Input: part model. Units: mm. Frame: model coordinates. Face numbers are marked on the shaded views. A direction names the side the tool comes from. Round coordinates to 2 decimals unless told otherwise and drop trailing zeros. Loops run counter-clockwise (first coordinate to the right, second up) from the corner with the lowest first, then second, coordinate; pieces in that order, holes last. Notation, with made-up numbers: (83, 77.25) -> (112, 77.25) arc R19 ccw to (112, 86.25) -> close; hole circle Ø6 at (39.5, -27). An arc over 180 degrees is marked (long way). One line per question, with ' | ' between items. Start each with the question number.
Q1. Cut plane D-D on y = 58. Return loops of the section in (x, z).
Q2. Cut plane C-C on z = 4.75. State how many separate pieces and enclosed holes the cut face has, and give its area (3 significant figures).
Q3. Cut plane A-A on x = -30. Return loops of the section in (y, z), and give its area (3 significant figures).
Q4. Access query for the marked faces 1, 2 and 3. Directions: +Z, -Z, +X, -X, +Y, -Y. A direction counts if a zero-diameter tool reaches every point of the face in a straight line with its end or side. Return the directions, or none.
Q5. Material intervals for L1, parallel to Y at x = 30, z = 4.25; L2, parallel to Y at x = -40, z = 3.25; L3, parallel to Y at x = 54.5, z = 4.5, sorted ascending.
Q6. Cut plane B-B on x = -15. Return loops of the section in (y, z), and give its area (3 significant figures).
Q7. Mould query, pull axis Y, two halves, no side actions, for the marked faces 4, 5 and 6. Classes: pulls with the +Y half, pulls with the -Y half, needs draft (parallel to the pull), parting line crosses it, or undercut.
Q8. Contact query for a flat-ended pin moving along its axis: P1, Ø2, axis at x = 57.5, z = 3.5, coming from the +Y side. Output: stop coordinate, or through.
from build123d import *

# Parameters (mm, degrees)
BOSS_EXTRU_1_DEPTH      = 8
ESQUISSE2_R             = 2.5
ENL_V_MAT_EXTRU_1_DEPTH = 96.859271852
ENL_V_MAT_EXTRU_4_DEPTH = 96.859271852
ESQUISSE5_R             = 2.5
ENL_V_MAT_EXTRU_5_DEPTH = 96.859271852
ENL_V_MAT_EXTRU_6_DEPTH = 96.859271852


with BuildPart() as part:
    # Esquisse1 → Boss.-Extru.1 (new body)
    with BuildSketch(Plane.XY):
        with BuildLine():
            Line((65, 4), (65, 41))
            ThreePointArc((65, 41), (63.828427125, 43.828427125), (61, 45))
            Line((61, 45), (54, 45))
            ThreePointArc((54, 45), (51.171572875, 46.171572875), (50, 49))
            Line((50, 49), (50, 66))
            ThreePointArc((50, 66), (48.828427125, 68.828427125), (46, 70))
            Line((46, 70), (-46, 70))
            ThreePointArc((-46, 70), (-48.828427125, 68.828427125), (-50, 66))
            Line((-50, 66), (-50, 49))
            ThreePointArc((-50, 49), (-51.171572875, 46.171572875), (-54, 45))
            Line((-54, 45), (-61, 45))
            ThreePointArc((-61, 45), (-63.828427125, 43.828427125), (-65, 41))
            Line((-65, 41), (-65, 4))
            ThreePointArc((-65, 4), (-63.828427125, 1.171572875), (-61, 0))
            Line((-61, 0), (61, 0))
            ThreePointArc((61, 0), (63.828427125, 1.171572875), (65, 4))
        make_face()
    extrude(amount=BOSS_EXTRU_1_DEPTH)

    # Esquisse2 → Enlèv. mat.-Extru.1 (cut, through all)
    with BuildSketch(Plane.XY.offset(8)):
        with Locations((30, 50)):
            Circle(ESQUISSE2_R)
        with Locations(Location((-30, 50, 0), (0, 0, 180))):
            Circle(ESQUISSE2_R)
    extrude(amount=-ENL_V_MAT_EXTRU_1_DEPTH, mode=Mode.SUBTRACT)

    # Esquisse4 → Enlèv. mat.-Extru.4 (cut, through all)
    with BuildSketch(Plane.XY.offset(8)):
        with BuildLine():
            Line((-41, 45), (-10.363961031, 45))
            ThreePointArc((-10.363961031, 45), (-8.978141732, 44.074025149), (-9.303300859, 42.439339828))
            Line((-9.303300859, 42.439339828), (-20.863961031, 30.878679656))
            ThreePointArc((-20.863961031, 30.878679656), (-21.837231077, 30.228361402), (-22.985281374, 30))
            Line((-22.985281374, 30), (-41, 30))
            ThreePointArc((-41, 30), (-42.060660172, 30.439339828), (-42.5, 31.5))
            Line((-42.5, 31.5), (-42.5, 43.5))
            ThreePointArc((-42.5, 43.5), (-42.060660172, 44.560660172), (-41, 45))
        make_face()
        with BuildLine():
            Line((-41, 12), (-10.363961031, 12))
            ThreePointArc((-10.363961031, 12), (-8.978141732, 12.925974851), (-9.303300859, 14.560660172))
            Line((-9.303300859, 14.560660172), (-20.863961031, 26.121320344))
            ThreePointArc((-20.863961031, 26.121320344), (-21.837231077, 26.771638598), (-22.985281374, 27))
            Line((-22.985281374, 27), (-41, 27))
            ThreePointArc((-41, 27), (-42.060660172, 26.560660172), (-42.5, 25.5))
            Line((-42.5, 25.5), (-42.5, 13.5))
            ThreePointArc((-42.5, 13.5), (-42.060660172, 12.439339828), (-41, 12))
        make_face()
        with BuildLine():
            Line((42.5, 43.5), (42.5, 31.5))
            ThreePointArc((42.5, 31.5), (42.060660172, 30.439339828), (41, 30))
            Line((41, 30), (22.985281374, 30))
            ThreePointArc((22.985281374, 30), (21.837231077, 30.228361402), (20.863961031, 30.878679656))
            Line((20.863961031, 30.878679656), (9.303300859, 42.439339828))
            ThreePointArc((9.303300859, 42.439339828), (8.978141732, 44.074025149), (10.363961031, 45))
            Line((10.363961031, 45), (41, 45))
            ThreePointArc((41, 45), (42.060660172, 44.560660172), (42.5, 43.5))
        make_face()
        with BuildLine():
            Line((22.985281374, 27), (41, 27))
            ThreePointArc((41, 27), (42.060660172, 26.560660172), (42.5, 25.5))
            Line((42.5, 25.5), (42.5, 13.5))
            ThreePointArc((42.5, 13.5), (42.060660172, 12.439339828), (41, 12))
            Line((41, 12), (10.363961031, 12))
            ThreePointArc((10.363961031, 12), (8.978141732, 12.925974851), (9.303300859, 14.560660172))
            Line((9.303300859, 14.560660172), (20.863961031, 26.121320344))
            ThreePointArc((20.863961031, 26.121320344), (21.837231077, 26.771638598), (22.985281374, 27))
        make_face()
        with BuildLine():
            Line((-3.378679656, 44.121320344), (-16.878679656, 30.621320344))
            ThreePointArc((-16.878679656, 30.621320344), (-17.757359313, 28.5), (-16.878679656, 26.378679656))
            Line((-16.878679656, 26.378679656), (-3.378679656, 12.878679656))
            ThreePointArc((-3.378679656, 12.878679656), (-2.40540961, 12.228361402), (-1.257359313, 12))
            Line((-1.257359313, 12), (1.257359313, 12))
            ThreePointArc((1.257359313, 12), (2.40540961, 12.228361402), (3.378679656, 12.878679656))
            Line((3.378679656, 12.878679656), (16.878679656, 26.378679656))
            ThreePointArc((16.878679656, 26.378679656), (17.757359313, 28.5), (16.878679656, 30.621320344))
            Line((16.878679656, 30.621320344), (3.378679656, 44.121320344))
            ThreePointArc((3.378679656, 44.121320344), (2.40540961, 44.771638598), (1.257359313, 45))
            Line((1.257359313, 45), (-1.257359313, 45))
            ThreePointArc((-1.257359313, 45), (-2.40540961, 44.771638598), (-3.378679656, 44.121320344))
        make_face()
    extrude(amount=-ENL_V_MAT_EXTRU_4_DEPTH, mode=Mode.SUBTRACT)

    # Esquisse5 → Enlèv. mat.-Extru.5 (cut, through all)
    with BuildSketch(Plane.XY.offset(8)):
        with Locations((-45, 4)):
            Circle(ESQUISSE5_R)
        with Locations((-15, 4)):
            Circle(ESQUISSE5_R)
        with Locations((15, 4)):
            Circle(ESQUISSE5_R)
        with Locations((45, 4)):
            Circle(ESQUISSE5_R)
    extrude(amount=-ENL_V_MAT_EXTRU_5_DEPTH, mode=Mode.SUBTRACT)

    # Esquisse6 → Enlèv. mat.-Extru.6 (cut, through all)
    with BuildSketch(Plane.XY.offset(8)):
        with BuildLine():
            Line((57, 27.053539967), (57, 24.053539967))
            ThreePointArc((57, 24.053539967), (55, 22.053539967), (53, 24.053539967))
            Line((53, 24.053539967), (53, 27.053539967))
            ThreePointArc((53, 27.053539967), (55, 29.053539967), (57, 27.053539967))
        make_face()
        with BuildLine():
            Line((57, 34.053539967), (57, 37.053539967))
            ThreePointArc((57, 37.053539967), (55, 39.053539967), (53, 37.053539967))
            Line((53, 37.053539967), (53, 34.053539967))
            ThreePointArc((53, 34.053539967), (55, 32.053539967), (57, 34.053539967))
        make_face()
        with BuildLine():
            Line((-57, 34.053539967), (-57, 37.053539967))
            ThreePointArc((-57, 37.053539967), (-55, 39.053539967), (-53, 37.053539967))
            Line((-53, 37.053539967), (-53, 34.053539967))
            ThreePointArc((-53, 34.053539967), (-55, 32.053539967), (-57, 34.053539967))
        make_face()
        with BuildLine():
            Line((-57, 27.053539967), (-57, 24.053539967))
            ThreePointArc((-57, 24.053539967), (-55, 22.053539967), (-53, 24.053539967))
            Line((-53, 24.053539967), (-53, 27.053539967))
            ThreePointArc((-53, 27.053539967), (-55, 29.053539967), (-57, 27.053539967))
        make_face()
    extrude(amount=-ENL_V_MAT_EXTRU_6_DEPTH, mode=Mode.SUBTRACT)


solid = part.part
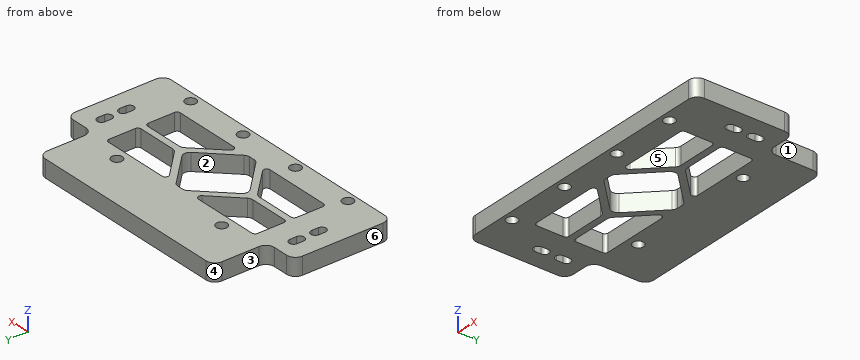
Results:
1) outline: (-50, 0) -> (50, 0) -> (50, 8) -> (-50, 8) -> close
2) separate pieces: 1 | enclosed holes: 15 | area: 5,740 mm^2
3) outline: (0, 0) -> (12, 0) -> (12, 8) -> (0, 8) -> close; (27, 0) -> (30, 0) -> (30, 8) -> (27, 8) -> close; (45, 0) -> (47.5, 0) -> (47.5, 8) -> (45, 8) -> close; (52.5, 0) -> (70, 0) -> (70, 8) -> (52.5, 8) -> close | area: 280 mm^2
4) face 1: +Z, -Z, +X, +Y | face 2: +Z, -Z | face 3: +Z, -Z, -X, +Y
5) L1: 0 to 12, 27 to 30, 45 to 47.5, 52.5 to 70 | L2: 0 to 12, 27 to 30, 45 to 70 | L3: 0 to 22.12, 28.99 to 32.12, 38.99 to 45
6) outline: (0, 0) -> (1.5, 0) -> (1.5, 8) -> (0, 8) -> close; (6.5, 0) -> (12, 0) -> (12, 8) -> (6.5, 8) -> close; (20.26, 0) -> (24.5, 0) -> (24.5, 8) -> (20.26, 8) -> close; (32.5, 0) -> (36.74, 0) -> (36.74, 8) -> (32.5, 8) -> close; (45, 0) -> (70, 0) -> (70, 8) -> (45, 8) -> close | area: 324 mm^2
7) face 4: pulls with the +Y half | face 5: undercut | face 6: needs draft
8) P1: y = 45
